Source: CAD feature listing. Evaluate the final solid. Frame: model axes, mm. Round coordinates to 2 decimals unless told otherwise and drop trailing zeros. Loops run counter-clockwise (first coordinate to the right, second up) from the corner with the lowest first, then second, coordinate; pieces in that order, holes last. Notation, with made-up numbers: (-33.75, 79.25) - (-11.75, 79.25) arc R30 cw to (-11.75, 112.25) - close; hole circle Ø10 at (-35, -38.5). An arc over 180 degrees is marked (long way). Use CSV: the item, a comma, the result in double quotes. Start each with the question number.
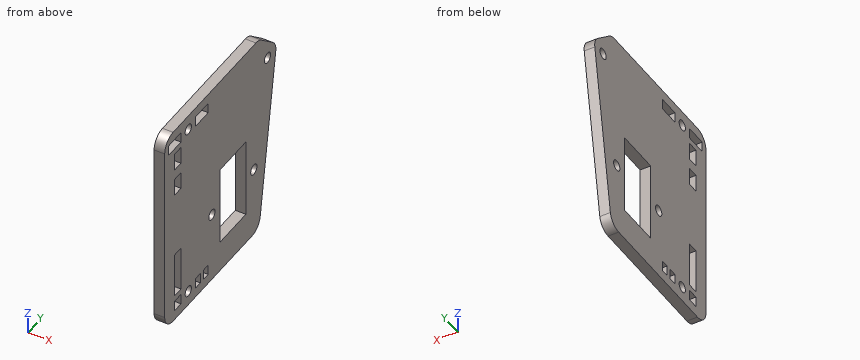
from build123d import *

# Parameters (mm, degrees)
RESSALTO_EXTRUS_O1_DEPTH   = 3
PERFIL_CORTE_W             = 23
PERFIL_CORTE_H             = 12.4
CORTE_PRINCIPAL_DEPTH      = 55.998187902
FURO_DE_DI_METRO_3_0_3_1_D = 3
ESBO_O6_W                  = 3
ESBO_O6_H                  = 6
ESBO_O6_H_2                = 2.25
ESBO_O6_H_3                = 3
CORTE_EXTRUS_O1_DEPTH      = 81.112421009
FURO_DE_DI_METRO_3_0_3_2_D = 3
FURO_DE_DI_METRO_3_0_3_3_D = 3
ESBO_O9_W                  = 5
ESBO_O9_H                  = 3
ESBO_O9_W_2                = 13
CORTE_EXTRUS_O2_DEPTH      = 81.112421009
FILETE1_R                  = 4


with BuildPart() as part:
    # Esboço1 → Ressalto-extrusão1 (new body)
    with BuildSketch(Plane(origin=(0, 0, 0), x_dir=(0, 0, -1), z_dir=(1, 0, 0))):
        with BuildLine():
            Line((0, 0), (60, 0))
            Line((60, 0), (60, 45))
            Line((60, 45), (9.320012162, 52.951655972))
            ThreePointArc((9.320012162, 52.951655972), (7.316640593, 52.753174223), (5.663681972, 51.603991711))
            Line((5.663681972, 51.603991711), (0, 45))
            Line((0, 45), (0, 0))
        make_face()
    extrude(amount=RESSALTO_EXTRUS_O1_DEPTH)

    # Perfil Corte → Corte Principal (cut, through all)
    with BuildSketch(Plane(origin=(0, 41.400449156, -36.080513885), x_dir=(0, 0, 1), z_dir=(-1, 0, 0))):
        with Locations((-3.419486115, -8.900449156)):
            Rectangle(PERFIL_CORTE_W, PERFIL_CORTE_H)
    extrude(amount=-CORTE_PRINCIPAL_DEPTH, mode=Mode.SUBTRACT)

    # Furo de diâmetro Ø3.0 (3)1 (through all)
    with Locations(Plane(origin=(0, -50, -154.479871529), x_dir=(0, 0, 1), z_dir=(-1, 0, 0))):
        with Locations((114.979871529, 92.5), (114.979871529, 72.5)):
            Hole(FURO_DE_DI_METRO_3_0_3_1_D / 2)

    # Esboço6 → Corte-extrusão1 (cut, through all)
    with BuildSketch(Plane(origin=(0, 0, 0), x_dir=(0, 0, -1), z_dir=(1, 0, 0))):
        with Locations((4.3, 17.75)):
            Rectangle(ESBO_O6_W, ESBO_O6_H)
        with Locations((4.3, 4.75)):
            Rectangle(ESBO_O6_W, ESBO_O6_H)
        with Locations((55.7, 19.625)):
            Rectangle(ESBO_O6_W, ESBO_O6_H_2)
        with Locations((55.7, 15.875)):
            Rectangle(ESBO_O6_W, ESBO_O6_H_2)
        with Locations((55.7, 6.25)):
            Rectangle(ESBO_O6_W, ESBO_O6_H_3)
    extrude(amount=CORTE_EXTRUS_O1_DEPTH, mode=Mode.SUBTRACT)

    # Furo de diâmetro Ø3.0 (3)2 (through all)
    with Locations(Plane(origin=(3, 0, 0), x_dir=(0, 0, -1), z_dir=(1, 0, 0))):
        with Locations((4.3, 11.25), (55.7, 11.25)):
            Hole(FURO_DE_DI_METRO_3_0_3_2_D / 2)

    # Furo de diâmetro Ø3.0 (3)3 (through all)
    with Locations(Plane.ZY):
        with Locations((-8.7, 49)):
            Hole(FURO_DE_DI_METRO_3_0_3_3_D / 2)

    # Esboço9 → Corte-extrusão2 (cut, through all)
    with BuildSketch(Plane(origin=(0, 0, 0), x_dir=(0, 0, -1), z_dir=(1, 0, 0))):
        with Locations((10, 6.25)):
            Rectangle(ESBO_O9_W, ESBO_O9_H)
        with Locations((18, 6.25)):
            Rectangle(ESBO_O9_W, ESBO_O9_H)
        with Locations((46, 6.25)):
            Rectangle(ESBO_O9_W_2, ESBO_O9_H)
    extrude(amount=CORTE_EXTRUS_O2_DEPTH, mode=Mode.SUBTRACT)

    # Filete1
    filete1_edges = [part.edges().sort_by_distance(p)[0] for p in [
        (1.5, 45, 0),
        (1.5, 45, -60),
        (1.5, 0, -60),
        (1.5, 0, 0),
    ]]
    fillet(filete1_edges, radius=FILETE1_R)


solid = part.part
1. Section query D-D on z = -18. Return the cut outline in (x, y).
2. Line query: line 1 along Z through (x, y) = (0.3, 19.5); line 2 along Y through (x, z) = (1.75, -8.7); line 3 along Z through (x, y) = (1.7, 32). Output: solid intervals per line, ascending.
3. Section query B-B on y = 22.5. Return the cut outline in (x, z), and give its area (3 significant figures).
4. Section query C-C on z = -47. Return the cut outline in (x, y), and give its area (3 significant figures).
5. Section query A-A on y = 11.25. Return the cut outline in (x, z), and give its area (3 significant figures).
6. Contact query for flat-ended pins moving along their axis: P1, Ø0.9, axis at x = 2, z = -55.5, coming from the +Y side; P2, Ø4, axis at y = 11.25, z = -4.3, coming from the -X side. Output: stop coordinate, or through.
Values:
1,outline,"(0, 0) - (3, 0) - (3, 4.75) - (0, 4.75) - close; (0, 7.75) - (3, 7.75) - (3, 51.59) - (0, 51.59) - close"
2,line 1,"z = -60 to -57.2, -54.2 to -5.8, -2.8 to 0"
2,line 2,"y = 0 to 4.75, 7.75 to 47.5, 50.5 to 53"
2,line 3,"z = -60 to -51, -28 to 0"
3,outline,"(0, -60) - (3, -60) - (3, -41) - (0, -41) - close; (0, -38) - (3, -38) - (3, 0) - (0, 0) - close"
3,area,"171 mm^2"
4,outline,"(0, 0) - (3, 0) - (3, 4.75) - (0, 4.75) - close; (0, 7.75) - (3, 7.75) - (3, 26.3) - (0, 26.3) - close; (0, 38.7) - (3, 38.7) - (3, 47.04) - (0, 47.04) - close"
4,area,"94.9 mm^2"
5,outline,"(0, -60) - (3, -60) - (3, -57.2) - (0, -57.2) - close; (0, -54.2) - (3, -54.2) - (3, -5.8) - (0, -5.8) - close; (0, -2.8) - (3, -2.8) - (3, 0) - (0, 0) - close"
5,area,"162 mm^2"
6,P1,"stops at y = 45.78"
6,P2,"stops at x = 0"
